Geometry: final body of the model. Coordinates: model frame, mm. A direction names the side the tool comes from. Coordinates: 2 decimals unless noted, no trailing zeros. Loops run counter-clockwise (first coordinate to the right, second up) from the corner with the lowest first, then second, coordinate; pieces in that order, holes last. Notation, with made-up numbers: (55, 77.5) - (112, 77.5) arc R24 cw to (112, 103.5) - close; hole circle Ø3 at (70, 36.5). An arc over 180 degrees is marked (long way). Write each question's results on one line, items separated by ' | '. Start each with the question number.
from build123d import *

# Parameters (mm, degrees)
F1_DEPTH = 25.4
F2_R     = 3.175
F3_DEPTH = 25.4
F4_R     = 3.175
F5_DEPTH = 25.4


with BuildPart() as f1:
    # F0 (on Front) → F1 (new body)
    with BuildSketch(Plane.XZ):
        Polygon((0, 25.4), (0, 0), (25.4, 0), (25.4, 3.175), (3.175, 3.175), (3.175, 25.4), align=None)
    extrude(amount=F1_DEPTH)

    # F2 (on face) → F3 (cut)
    with BuildSketch(Plane(origin=(0, 0, 0), x_dir=(0, -1, 0), z_dir=(-1, 0, 0))):
        with Locations((6.35, 12.7)):
            Circle(F2_R)
        with Locations((19.05, 12.7)):
            Circle(F2_R)
    extrude(amount=-F3_DEPTH, mode=Mode.SUBTRACT)

    # F4 (on face) → F5 (cut)
    with BuildSketch(Plane(origin=(0, 0, 0), x_dir=(1, 0, 0), z_dir=(0, 0, -1))):
        with Locations((12.7, 19.05)):
            Circle(F4_R)
        with Locations((12.7, 6.35)):
            Circle(F4_R)
    extrude(amount=-F5_DEPTH, mode=Mode.SUBTRACT)


solid = f1.part
1) Pull-direction query (Y, two-part tool) for faces 1 (the flat face through (7, 0, 2)), 2 (the flat face through (3.175, -13, 14)), 3 (the cylindrical face through (1.57, -3.83, 10.77)); classes: released by +Y, released by -Y, zero draft, split by the parting line, or undercut.
2) Pin query (flat end, axial travel): pin 1 Ø10 at (y, z) = (-19.05, 12.7) entering from +X (3 decimals); pin 2 Ø12 at (x, z) = (12.5, 8) entering from +Y; pin 3 Ø8.5 at (x, y) = (12.7, -6.35) entering from +Z (3 decimals); pin 4 Ø4 at (x, z) = (6, 7) entering from +Y. Return the tip coordinate at first contact, or that it passes through.
3) Section query B-B on y = -19.05. Output: boundary loops of the cut face in (x, z) (3 decimals), and give its area (3 significant figures).
4) Section query D-D on z = 2. Output: boundary loops of the cut face in (x, y) (3 decimals), and give its area (3 significant figures).
5) Section query C-C on x = 12.7. Output: boundary loops of the cut face in (y, z) (3 decimals), and give its area (3 significant figures).
6) Material intervals for line 1 (Y direction, x = 12.7, z = 1.6) (3 decimals); line 2 (X direction, y = -6.35, z = 2.3) (3 decimals), sorted ascending. Write a range as [from, to].
7) Section query A-A on z = 12.7. Output: boundary loops of the cut face in (x, y) (3 decimals).
8) Access query for faces 4 (the flat face through (25.4, -13, 2)), 5 (the flat face through (14, -13, 3.175)). Directions: +Z, -Z, +X, -X, +Y, -Y. A direction counts if a zero-diameter tool reaches every point of the face in a straight line with its end or side. Return the directions, or none.
Returned:
1) face 1: released by +Y | face 2: zero draft | face 3: undercut
2) pin 1: stops at x = 3.175 | pin 2: stops at y = 0 | pin 3: stops at z = 3.175 | pin 4: passes through
3) outline: (0, 0) - (9.525, 0) - (9.525, 3.175) - (3.175, 3.175) - (3.175, 9.525) - (0, 9.525) - close; (0, 15.875) - (3.175, 15.875) - (3.175, 25.4) - (0, 25.4) - close; (15.875, 0) - (25.4, 0) - (25.4, 3.175) - (15.875, 3.175) - close | area: 111 mm²
4) outline: (0, -25.4) - (25.4, -25.4) - (25.4, 0) - (0, 0) - close; hole circle Ø6.35 at (12.7, -19.05); hole circle Ø6.35 at (12.7, -6.35) | area: 582 mm²
5) outline: (-25.4, 0) - (-22.225, 0) - (-22.225, 3.175) - (-25.4, 3.175) - close; (-15.875, 0) - (-9.525, 0) - (-9.525, 3.175) - (-15.875, 3.175) - close; (-3.175, 0) - (0, 0) - (0, 3.175) - (-3.175, 3.175) - close | area: 40.3 mm²
6) line 1: y = [-25.4, -22.225], [-15.875, -9.525], [-3.175, 0] | line 2: x = [0, 9.525], [15.875, 25.4]
7) outline: (0, -25.4) - (3.175, -25.4) - (3.175, -22.225) - (0, -22.225) - close; (0, -15.875) - (3.175, -15.875) - (3.175, -9.525) - (0, -9.525) - close; (0, -3.175) - (3.175, -3.175) - (3.175, 0) - (0, 0) - close
8) face 4: +Z, -Z, +X, +Y, -Y | face 5: +Z, +X, +Y, -Y
